from build123d import *

# Parameters (mm, degrees)
SKETCH1_R           = 2.5
BOSS_EXTRUDE1_DEPTH = 20
SKETCH2_R           = 3.5
BOSS_EXTRUDE2_DEPTH = 1
CHAMFER1_SIZE       = 0.5


with BuildPart() as part:
    # Sketch1 → Boss-Extrude1 (new body, symmetric)
    with BuildSketch(Plane.XY):
        Circle(SKETCH1_R)
    extrude(amount=BOSS_EXTRUDE1_DEPTH, both=True)

    # Sketch2 → Boss-Extrude2 (add)
    with BuildSketch(Plane.XY.offset(20)):
        Circle(SKETCH2_R)
    boss_extrude2 = extrude(amount=BOSS_EXTRUDE2_DEPTH)

    # Mirror1: Boss-Extrude2 across plane
    add(boss_extrude2.mirror(Plane.XY))

    # Chamfer1
    chamfer1_edges = [part.edges().sort_by_distance(p)[0] for p in [
        (-3.5, 0, 21),
        (-3.5, 0, -21),
    ]]
    chamfer(chamfer1_edges, length=CHAMFER1_SIZE)


solid = part.part
Design review of the part built by this model. Coordinates are the model's own, in mm. A direction names the side the tool comes from. Give positions to 0.01 mm unless a question says otherwise; leave off trailing zeros. Order: outer loops, then holes, each group sorted by start corner. A loop starts at its lowest first (then second) coordinate and runs counter-clockwise, first axis right, second up. Notation, with made-up numbers: (60.25, 2) - (71.25, 2) arc R26 ccw to (71.25, 41) - close; hole circle Ø11 at (-5.75, -27.5). An arc over 180 degrees is marked (long way). Write item = value, one per line. Start each with the question number.
Q1. We need section A-A on x = 0. State the section outline as (y, z) points.
Q2. To check wall thickness, follow L1, parallel to Z at x = 2.75, y = -0.75; L2, parallel to Z at x = -2.75, y = -2; L3, parallel to Y at x = 0, z = -4. State the ranges of each line that lie inside material, in increasing order. Write a range as from..to.
Q3. Mouldability with a two-part tool opening along Z and no side actions: class faces 1 (the face through (2, -2, -20)), 2 (the face through (0, 0, -21)), 3 (the face through (3.233, -1.341, 20.246)) as released by +Z, released by -Z, zero draft, split by the parting line, or undercut.
Q4. Clearance check with flat-ended pins moving along their axes: pin 1 Ø3 at (x, z) = (-2.5, 10) entering from -Y; pin 2 Ø1.5 at (y, z) = (-2, -12) entering from -X. State where each tip first meets the part, or that it passes through.
Q5. We need section C-C on z = -14. State the section outline as (x, y) points, plus the area to 3 significant figures.
Q6. Tool access review of faces 4 (the face through (-0.54, -2.44, 0.28)), 5 (the face through (3.233, -1.341, -20.246)): name each direction out of +Z, -Z, +X, -X, +Y, -Y from which nothing blocks a thin tool from reaching the whole face with its end or side.
Working result:
q1.outline = (-3.5, -20.5) - (-3, -21) - (3, -21) - (3.5, -20.5) - (3.5, -20) - (2.5, -20) - (2.5, 20) - (3.5, 20) - (3.5, 20.5) - (3, 21) - (-3, 21) - (-3.5, 20.5) - (-3.5, 20) - (-2.5, 20) - (-2.5, -20) - (-3.5, -20) - close
q2.L1 = -21..-20, 20..21
q2.L2 = -20.6..-20, 20..20.6
q2.L3 = -2.5..2.5
q3.face_1 = undercut
q3.face_2 = released by -Z
q3.face_3 = zero draft
q4.pin_1 = -2.29
q4.pin_2 = -2.17
q5.outline = circle Ø5 at (0, 0)
q5.area = 19.6 mm²
q6.face_4 = none
q6.face_5 = +Z, -Z
